from build123d import *

# Parameters (mm, degrees)
F1_DEPTH = 8
F2_R     = 2
F4_DEPTH = 4


with BuildPart() as f1:
    # F0 (on Top) → F1 (new body)
    with BuildSketch(Plane.XY):
        with BuildLine():
            Line((-15, -40), (15, -40))
            ThreePointArc((15, -40), (22.071068, -37.071068), (25, -30))
            Line((25, -30), (25, 30))
            ThreePointArc((25, 30), (22.071068, 37.071068), (15, 40))
            Line((15, 40), (-15, 40))
            ThreePointArc((-15, 40), (-22.071068, 37.071068), (-25, 30))
            Line((-25, 30), (-25, -30))
            ThreePointArc((-25, -30), (-22.071068, -37.071068), (-15, -40))
        make_face()
    extrude(amount=F1_DEPTH)

    # F2
    f2_edges = [f1.edges().sort_by_distance(p)[0] for p in [
        (0, -40, 8),
        (22.071068, -37.071068, 8),
        (25, 0, 8),
        (22.071068, 37.071068, 8),
        (0, 40, 8),
        (-22.071068, 37.071068, 8),
        (-25, 0, 8),
        (-22.071068, -37.071068, 8),
    ]]
    fillet(f2_edges, radius=F2_R)

    # F3 (on face) → F4 (cut)
    with BuildSketch(Plane.XY.offset(8)):
        with BuildLine():
            Line((-10, -30), (10, -30))
            ThreePointArc((10, -30), (13.535534, -28.535534), (15, -25))
            Line((15, -25), (15, 25))
            ThreePointArc((15, 25), (13.535534, 28.535534), (10, 30))
            Line((10, 30), (-10, 30))
            ThreePointArc((-10, 30), (-13.535534, 28.535534), (-15, 25))
            Line((-15, 25), (-15, -25))
            ThreePointArc((-15, -25), (-13.535534, -28.535534), (-10, -30))
        make_face()
    extrude(amount=-F4_DEPTH, mode=Mode.SUBTRACT)


solid = f1.part
Could you check a few things on this model? Use its own coordinates, in mm. A direction names the side the tool comes from. Give positions to 0.01 mm unless a question says otherwise; leave off trailing zeros. Order: outer loops, then holes, each group sorted by start corner. A loop starts at its lowest first (then second) coordinate and runs counter-clockwise, first axis right, second up. Notation, with made-up numbers: (-24.75, 27) - (29.25, 27) arc R22 ccw to (29.25, 65) - close; hole circle Ø11 at (-8, 16). An arc over 180 degrees is marked (long way). One line per question, with ' | ' between items. Start each with the question number.
Item 1: Thinking about a two-plate mould opening in X: for faces 3 (the flat face through (0, 0, 4)), 4 (the flat face through (15, 0, 6)), 5 (the flat face through (0, 1, 0)), 6 (the cylindrical face through (-22.15, -36.99, 2.96)), which applies, pulls with the +X half, pulls with the -X half, needs draft (parallel to the pull), parting line crosses it, or undercut?
Item 2: I want a section at C-C on x = -5.5. Write out the boundary of the cut face in (y, z), then the cut area to 3 significant figures.
Item 3: I want a section at B-B on y = 3. Write out the boundary of the cut face in (x, z), then the cut area to 3 significant figures.
Item 4: I want a section at A-A on z = 5. Write out the boundary of the cut face in (x, y).
Item 5: I need wall thicknesses on probe 1 along X at (y, z) = (-23.5, 4.75); probe 2 along Y at (x, z) = (9.5, 5.25); probe 3 along Y at (x, z) = (-3, 7). Which ranges of each line are inside material? Lowest first, please. Write a range as [from, to].
Item 6: I'm going to push flat-ended pins straight in: pin 1 Ø1.5 at (x, z) = (16, 3.5) entering from -Y; pin 2 Ø4 at (x, z) = (20, 6.5) entering from -Y. Where does each tip first touch, or does it pass through?
Item 7: For faces 1 (the cylindrical face through (-13, 29, 6)), 2 (the cylindrical face through (-0.21, 39.43, 7.4)), which set-ups out of +Z, -Z, +X, -X, +Y, -Y let a thin tool reach every point of the face, with its end or its side?
Verdict:
1) face 3: undercut | face 4: undercut | face 5: needs draft | face 6: pulls with the -X half
2) outline: (-40, 0) - (40, 0) - (40, 6) arc R2 ccw to (38, 8) - (30, 8) - (30, 4) - (-30, 4) - (-30, 8) - (-38, 8) arc R2 ccw to (-40, 6) - close | area: 398 mm^2
3) outline: (-25, 0) - (25, 0) - (25, 6) arc R2 ccw to (23, 8) - (15, 8) - (15, 4) - (-15, 4) - (-15, 8) - (-23, 8) arc R2 ccw to (-25, 6) - close | area: 278 mm^2
4) outline: (-25, -30) arc R10 ccw to (-15, -40) - (15, -40) arc R10 ccw to (25, -30) - (25, 30) arc R10 ccw to (15, 40) - (-15, 40) arc R10 ccw to (-25, 30) - close; hole (-15, -25) arc R5 ccw to (-10, -30) - (10, -30) arc R5 ccw to (15, -25) - (15, 25) arc R5 ccw to (10, 30) - (-10, 30) arc R5 ccw to (-15, 25) - close
5) probe 1: [-25, -15], [15, 25] | probe 2: [-40, -30], [30, 40] | probe 3: [-39.73, -30], [30, 39.73]
6) pin 1: y = -40 | pin 2: y = -39.52
7) face 1: +Z | face 2: +Z, +X, -X, +Y
